Check sheet for the drawn part. Datum: minimum x, y, z corner. Units: mm. Round coordinates to 2 decimals unless told otherwise and drop trailing zeros. Write each loop counter-clockwise with the first axis right and the second up, starting at its lowest first coordinate (ties: lowest second). Pieces come first, ordered by that corner, then holes. Notation, with made-up numbers: M 81.25,-13 L 85.25,-13 A23 cw 85.25,-4 Z; hole C 24.25,-19 d9. An arc over 180 degrees is marked long. One line per item, written item: value.
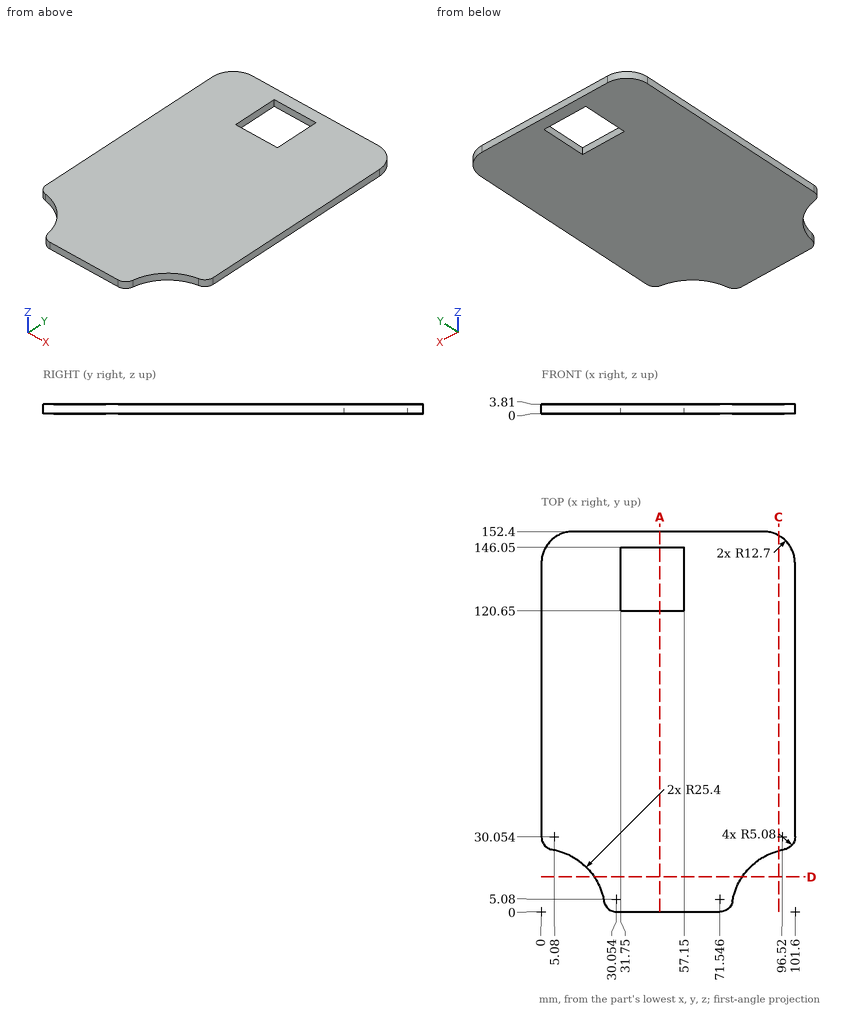
Q1. Sectioned sample at A-A on x = 47.5. Enter the section's corners in (y, z), and give its area (3 significant figures).
Completed:
outline: M 0,0 L 120.65,0 L 120.65,3.81 L 0,3.81 Z; M 146.05,0 L 152.4,0 L 152.4,3.81 L 146.05,3.81 Z
area: 484 mm^2
Q2. Sectioned sample at C-C on x = 95. Enter the section's corners in (y, z).
Completed:
outline: M 24.53,0 L 150.84,0 L 150.84,3.81 L 24.53,3.81 Z
Q3. Scan lines: line 1 (Y direction, x = 50, z = 3); line 2 (X direction, y = 146, z = 1.7); line 3 (X direction, y = 9, z = 3.65). Record each from-to range of solid material in increasing order. Write a range as [from, to].
Completed:
line 1: [0, 120.65], [146.05, 152.4]
line 2: [1.67, 31.75], [57.15, 99.93]
line 3: [23.75, 77.85]
Q4. Sectioned sample at D-D on y = 14. Enter the section's corners in (x, z), and give its area (3 significant figures).
Completed:
outline: M 21.19,0 L 80.41,0 L 80.41,3.81 L 21.19,3.81 Z
area: 226 mm^2
